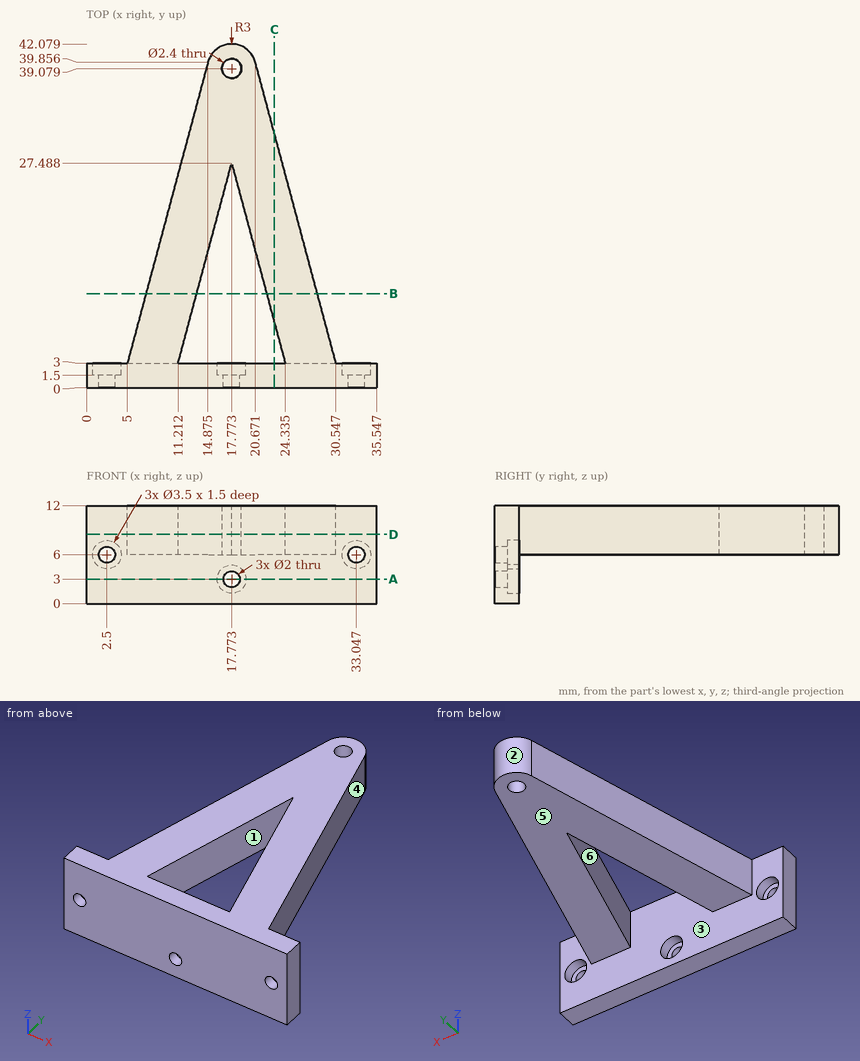
Part print with two shaded views. Sizes in mm from the minimum x, y, z corner. A direction names the side the tool comes from. Round coordinates to 2 decimals unless told otherwise and drop trailing zeros. Order: outer loops, then holes, each group sorted by start corner. A loop starts at its lowest first (then second) coordinate and runs counter-clockwise, first axis right, second up. Notation, with made-up numbers: M 56,-1 L 87,-1 A29 cw 87,26 Z; hole C 34,78.25 d9. An arc over 180 degrees is marked long. Put each result on its own line as item: value. Start each with the question number.
1. Slice it at B-B on y = 11.5. List the corners of the cut face in (x, z).
2. Tool access for the marked faces 1, 2 and 3: list every direction of +Z, -Z, +X, -X, +Y, -Y with a clear straight run to the whole face (end or side of a thin tool).
3. Slice it at D-D on z = 8.5. List the corners of the cut face in (x, y) (1 decimal).
4. Slice it at C-C on x = 23. List the corners of the cut face in (y, z).
5. Slice it at A-A on z = 3. List the corners of the cut face in (x, y).
6. Two-plate mould, pull along Y, no slides. Class the marked faces 4, 5 and 6: +Y half, -Y half, draft (parallel to the pull), parting line (faces both ways), or undercut.
7. Drill centre lines: probe 1 along X at (y, z) = (0.8, 6); probe 2 along Y at (x, z) = (31, 6.5); probe 3 along X at (y, z) = (0.95, 3). Where is each one in solid material? Low to high. Write a range as [from, to].
8. Drop flat-ended pins along their axis: pin 1 (5 mm diameter, centred on y = 14.5, z = 10.5, fed in from +X) (1 decimal); pin 2 (2.5 mm diameter, centred on x = 2.5, z = 6, fed in from +Y); pin 3 (5 mm diameter, centred on x = 23.5, y = 8, fed in from -Z). Give the stop position or say it passes through.
Findings:
1. outline: M 7.28,6 L 13.49,6 L 13.49,12 L 7.28,12 Z; M 22.06,6 L 28.27,6 L 28.27,12 L 22.06,12 Z
2. face 1: +Z, -Z
2. face 2: +Z, -Z, +Y
2. face 3: -Z
3. outline: M 0,0 L 35.5,0 L 35.5,3 L 30.5,3 L 20.7,39.9 A3 ccw 14.9,39.9 L 5,3 L 0,3 Z; hole M 11.2,3 L 24.3,3 L 17.8,27.5 Z; hole C 17.8,39.1 d2.4
4. outline: M 0,0 L 3,0 L 3,12 L 0,12 Z; M 7.98,6 L 31.16,6 L 31.16,12 L 7.98,12 Z
5. outline: M 0,0 L 16.77,0 L 16.77,1.5 L 16.02,1.5 L 16.02,3 L 0,3 Z; M 18.77,0 L 35.55,0 L 35.55,3 L 19.52,3 L 19.52,1.5 L 18.77,1.5 Z
6. face 4: +Y half
6. face 5: draft
6. face 6: undercut
7. probe 1: [0, 1.5], [3.5, 32.05], [34.05, 35.55]
7. probe 2: [0, 3]
7. probe 3: [0, 16.77], [18.77, 35.55]
8. pin 1: x = 28.1
8. pin 2: y = 1.5
8. pin 3: z = 6
